Check sheet for the modelled part. Datum: model origin and axes. Units: mm. A direction names the side the tool comes from. Round coordinates to 2 decimals unless told otherwise and drop trailing zeros. Write each loop counter-clockwise with the first axis right and the second up, starting at its lowest first coordinate (ties: lowest second). Pieces come first, ordered by that corner, then holes.
Item 1: Depth check by flat-ended pin: pin 1 (5 mm diameter, centred on y = 11.5, z = -2, fed in from -X); pin 2 (2 mm diameter, centred on x = -6.57, z = -3.55, fed in from +Y); pin 3 (5.5 mm diameter, centred on x = -5, z = 4, fed in from -Y); pin 4 (5 mm diameter, centred on y = 10, z = -10, fed in from +X). Enter the tip coordinate at first touch or a pass-through.
Item 2: Section check B-B, the plane y = 10.5. Record the cut outline in (x, z), plus the area to 3 significant figures.
Item 3: Section check A-A, the plane z = 25. Record the cut outline in (x, y), plus the area to 3 significant figures.
Item 4: Section check C-C, the plane x = -1.27. Record the cut outline in (y, z), plus the area to 3 significant figures.
Item 5: Release check for a two-part mould opening along X. For faces 6 (the flat face through (1, 4, 0)), 7 (the flat face through (16.437, 8, 0)), 8 (the flat face through (1, 8, 8.969)) record: pulls with the +X half, pulls with the -X half, needs draft (parallel to the pull), parting line crosses it, or undercut.
Item 6: Material ranges on line 1 along X through (y, z) = (0.7, 25); line 2 along X through (y, z) = (10.25, -5.05); line 3 along X through (y, z) = (12.25, -3.55), recorded low to high.
Item 7: Set-up check for faces 1 (the flat face through (15.297, 1, 22)), 2 (the flat face through (1, 8, -9.182)), 3 (the flat face through (-17.5, 1, 0)), 4 (the flat face through (1, 2, 8.83)), 5 (the flat face through (-12, 0, 0)): record each of +Z, -Z, +X, -X, +Y, -Y from which the full face is reachable in a straight line by a thin tool's end or side.
Item 8: Section check D-D, the plane y = 2.25. Record the cut outline in (x, z), plus the area to 3 significant figures.
from build123d import *

# Parameters (mm, degrees)
SKETCH1_W           = 35
SKETCH1_H           = 55
SKETCH1_R           = 1.5
SKETCH1_R_2         = 1.25
SKETCH1_W_2         = 1.053264104
SKETCH1_H_2         = 1.810086697
BOSS_EXTRUDE1_DEPTH = 3
SKETCH2_W           = 30.130506089
SKETCH2_H           = 18.151203477
BOSS_EXTRUDE2_DEPTH = 11
SKETCH3_R           = 1.25
CUT_EXTRUDE1_DEPTH  = 35.402034824
SKETCH4_W           = 25.972666726
SKETCH4_H           = 17.735623468
CUT_EXTRUDE2_DEPTH  = 4


with BuildPart() as part:
    # Sketch1 → Boss-Extrude1 (new body)
    with BuildSketch(Plane(origin=(0, 0, 0), x_dir=(1, 0, 0), z_dir=(0, 1, 0))):
        Rectangle(SKETCH1_W, SKETCH1_H)
        with Locations(Location((12.5, 25, 0), (0, 0, 270))):
            Circle(SKETCH1_R, mode=Mode.SUBTRACT)
        with Locations(Location((-12.5, 25, 0), (0, 0, 270))):
            Circle(SKETCH1_R, mode=Mode.SUBTRACT)
        with Locations(Location((12.5, -25, 0), (0, 0, 270))):
            Circle(SKETCH1_R, mode=Mode.SUBTRACT)
        with Locations(Location((-12.5, -25, 0), (0, 0, 270))):
            Circle(SKETCH1_R, mode=Mode.SUBTRACT)
        with Locations(Location((-1.27, -4.95, 0), (0, 0, 90))):
            Circle(SKETCH1_R_2, mode=Mode.SUBTRACT)
        with Locations(Location((-6.57, 3.55, 0), (0, 0, 90))):
            Circle(SKETCH1_R_2, mode=Mode.SUBTRACT)
        with Locations(Location((10.83, 5.05, 0), (0, 0, 90))):
            Circle(SKETCH1_R_2, mode=Mode.SUBTRACT)
        with Locations(Location((9.53, -3.55, 0), (0, 0, 90))):
            Circle(SKETCH1_R_2, mode=Mode.SUBTRACT)
        with Locations((14.770586435, -21.896230663)):
            Rectangle(SKETCH1_W_2, SKETCH1_H_2, mode=Mode.SUBTRACT)
    extrude(amount=BOSS_EXTRUDE1_DEPTH)

    # Sketch2 → Boss-Extrude2 (add)
    with BuildSketch(Plane(origin=(0, 3, 0), x_dir=(1, 0, 0), z_dir=(0, 1, 0))):
        with Locations((1.371677436, 0.106547158)):
            Rectangle(SKETCH2_W, SKETCH2_H)
    extrude(amount=BOSS_EXTRUDE2_DEPTH)

    # Sketch3 → Cut-Extrude1 (cut, through all)
    with BuildSketch(Plane.XZ.offset(-3)):
        with Locations(Location((-1.27, 4.95, 0), (0, 0, 270))):
            Circle(SKETCH3_R)
        with Locations(Location((-6.57, -3.55, 0), (0, 0, 270))):
            Circle(SKETCH3_R)
        with Locations(Location((9.53, 3.55, 0), (0, 0, 270))):
            Circle(SKETCH3_R)
        with Locations(Location((10.83, -5.05, 0), (0, 0, 270))):
            Circle(SKETCH3_R)
    extrude(amount=-CUT_EXTRUDE1_DEPTH, mode=Mode.SUBTRACT)

    # Sketch4 → Cut-Extrude2 (cut)
    with BuildSketch(Plane.XZ):
        with Locations((1.214862274, -0.038232514)):
            Rectangle(SKETCH4_W, SKETCH4_H)
    extrude(amount=-CUT_EXTRUDE2_DEPTH, mode=Mode.SUBTRACT)


solid = part.part
Values found:
1. pin 1: stops at x = -13.69
1. pin 2: passes through
1. pin 3: stops at y = 4
1. pin 4: stops at x = 16.44
2. outline: (-13.69, -9.18) - (16.44, -9.18) - (16.44, 8.97) - (-13.69, 8.97) - close; hole circle Ø2.5 at (-6.57, -3.55); hole circle Ø2.5 at (-1.27, 4.95); hole circle Ø2.5 at (9.53, 3.55); hole circle Ø2.5 at (10.83, -5.05)
2. area: 527 mm2
3. outline: (-17.5, 0) - (-14, 0) - (-14, 3) - (-17.5, 3) - close; (-11, 0) - (11, 0) - (11, 3) - (-11, 3) - close; (14, 0) - (17.5, 0) - (17.5, 3) - (14, 3) - close
3. area: 87.0 mm2
4. outline: (0, -27.5) - (3, -27.5) - (3, -9.18) - (14, -9.18) - (14, 3.7) - (4, 3.7) - (4, -8.91) - (0, -8.91) - close; (0, 8.83) - (4, 8.83) - (4, 6.2) - (14, 6.2) - (14, 8.97) - (3, 8.97) - (3, 27.5) - (0, 27.5) - close
4. area: 269 mm2
5. face 6: undercut
5. face 7: pulls with the +X half
5. face 8: needs draft
6. line 1: x = -17.5 to -14, -11 to 11, 14 to 17.5
6. line 2: x = -13.69 to 9.58, 12.08 to 16.44
6. line 3: x = -13.69 to -7.82, -5.32 to 16.44
7. face 1: +Y, -Y
7. face 2: -Z, +X, -X, +Y
7. face 3: +Z, -Z, -X, +Y, -Y
7. face 4: -Y
7. face 5: +Z, -Z, +X, -X, -Y
8. outline: (-17.5, -27.5) - (17.5, -27.5) - (17.5, 27.5) - (-17.5, 27.5) - close; hole circle Ø3 at (-12.5, -25); hole circle Ø3 at (-12.5, 25); hole (-11.77, -8.91) - (14.2, -8.91) - (14.2, 8.83) - (-11.77, 8.83) - close; hole circle Ø3 at (12.5, -25); hole circle Ø3 at (12.5, 25); hole (14.24, 20.99) - (15.3, 20.99) - (15.3, 22.8) - (14.24, 22.8) - close
8. area: 1,430 mm2
